Verification items for the finished model (mm, model axes). A direction names the side the tool comes from. Round coordinates to 2 decimals unless told otherwise and drop trailing zeros. Write each loop counter-clockwise with the first axis right and the second up, starting at its lowest first coordinate (ties: lowest second). Pieces come first, ordered by that corner, then holes.
from build123d import *

# Parameters (mm, degrees)
EXTRUDE_1_DEPTH     = 3
SKETCH_2_R          = 1.45
CUT_EXTRUDE_1_DEPTH = 3
SKETCH_3_W          = 50
SKETCH_3_H          = 3
EXTRUDE_2_DEPTH     = 8
SKETCH_4_W          = 50
SKETCH_4_H          = 5
EXTRUDE_3_DEPTH     = 16
SKETCH_6_W          = 27
SKETCH_6_H          = 5
EXTRUDE_4_DEPTH     = 7
SKETCH_7_R          = 1.45
CUT_EXTRUDE_2_DEPTH = 7
SKETCH_8_R          = 3
CUT_EXTRUDE_3_DEPTH = 2
FILLET_1_R          = 1
FILLET_2_R          = 2.5
SKETCH_9_R          = 1.45
CUT_EXTRUDE_4_DEPTH = 10


# Some blends are built 0.0001 mm under size
with BuildPart() as part:
    # Эскиз1 → Бобышка-Вытянуть1 (new body)
    with BuildSketch(Plane(origin=(0, 0, 0), x_dir=(1, 0, 0), z_dir=(0, 1, 0))):
        Polygon((-25, 0), (-12.5, 21.650635095), (12.5, 21.650635095), (25, 0), align=None)
    extrude(amount=EXTRUDE_1_DEPTH)

    # Эскиз2 → Вырез-Вытянуть1 (cut)
    with BuildSketch(Plane(origin=(0, 3, 0), x_dir=(1, 0, 0), z_dir=(0, 1, 0))):
        with Locations(Location((-10, 18.650635095, 0), (0, 0, 270))):
            Circle(SKETCH_2_R)
        with Locations(Location((-18, 4.794228634, 0), (0, 0, 270))):
            Circle(SKETCH_2_R)
        with Locations(Location((18, 4.794228634, 0), (0, 0, 90))):
            Circle(SKETCH_2_R)
        with Locations(Location((10, 18.650635095, 0), (0, 0, 90))):
            Circle(SKETCH_2_R)
        with Locations(Location((-6, 4.794228634, 0), (0, 0, 270))):
            Circle(SKETCH_2_R)
        with Locations(Location((6, 4.794228634, 0), (0, 0, 270))):
            Circle(SKETCH_2_R)
    extrude(amount=-CUT_EXTRUDE_1_DEPTH, mode=Mode.SUBTRACT)

    # Эскиз3 → Бобышка-Вытянуть2 (add)
    with BuildSketch(Plane.XY):
        with Locations((0, 1.5)):
            Rectangle(SKETCH_3_W, SKETCH_3_H)
    extrude(amount=EXTRUDE_2_DEPTH)

    # Эскиз4 → Бобышка-Вытянуть3 (add)
    with BuildSketch(Plane(origin=(0, 3, 0), x_dir=(1, 0, 0), z_dir=(0, 1, 0))):
        with Locations((0, -5.5)):
            Rectangle(SKETCH_4_W, SKETCH_4_H)
    extrude(amount=EXTRUDE_3_DEPTH)

    # Эскиз6 → Бобышка-Вытянуть4 (add)
    with BuildSketch(Plane.XY.offset(8)):
        with Locations((0, 3.5)):
            Rectangle(SKETCH_6_W, SKETCH_6_H)
    extrude(amount=EXTRUDE_4_DEPTH)

    # Эскиз7 → Вырез-Вытянуть2 (cut)
    with BuildSketch(Plane.XZ.offset(-1)):
        with Locations(Location((-8.5, 11.5, 0), (0, 0, 270))):
            Circle(SKETCH_7_R)
        with Locations(Location((8.5, 11.5, 0), (0, 0, 270))):
            Circle(SKETCH_7_R)
    extrude(amount=-CUT_EXTRUDE_2_DEPTH, mode=Mode.SUBTRACT)

    # Эскиз8 → Вырез-Вытянуть3 (cut)
    with BuildSketch(Plane.XZ.offset(-1)):
        with Locations(Location((-8.5, 11.5, 0), (0, 0, 270))):
            Circle(SKETCH_8_R)
        with Locations(Location((8.5, 11.5, 0), (0, 0, 270))):
            Circle(SKETCH_8_R)
    extrude(amount=-CUT_EXTRUDE_3_DEPTH, mode=Mode.SUBTRACT)

    # Скругление1
    fillet_1_edges = [part.edges().sort_by_distance(p)[0] for p in [
        (25, 9.5, 8),
        (-25, 9.5, 8),
        (0, 0, 8),
        (-25, 11, 3),
        (25, 11, 3),
    ]]
    fillet(fillet_1_edges, radius=FILLET_1_R - 0.0001)  # a hair under: the kernel refuses the full size

    # Скругление2
    # the kernel refuses this fillet: 2.5 mm, written as the material it takes off along each edge
    with BuildSketch(Plane(origin=(22.5, 2.5, 8), x_dir=(0, -1, 0), z_dir=(-1, 0, 0))) as fillet_2_piece_1:
        with BuildLine():
            CenterArc((1.5001, -0.9999), 0.9999, 0, 90)
            Line((2.5, -0.9999), (2.5, 0))
            Line((2.5, 0), (1.5001, 0))
        make_face()
    revolve(axis=Axis((22.5, 2.5, 8), (0, 0, 1)), revolution_arc=90, mode=Mode.SUBTRACT)
    with BuildSketch(Plane(origin=(-22.5, 2.5, 8), x_dir=(-1, 0, 0), z_dir=(0, 1, 0))) as fillet_2_piece_2:
        with BuildLine():
            CenterArc((1.5001, -0.9999), 0.9999, 0, 90)
            Line((2.5, -0.9999), (2.5, 0))
            Line((2.5, 0), (1.5001, 0))
        make_face()
    revolve(axis=Axis((-22.5, 2.5, 8), (0, 0, 1)), revolution_arc=90, mode=Mode.SUBTRACT)
    with BuildSketch(Plane(origin=(25, 0, -6.25), x_dir=(0, 1, 0), z_dir=(0, 0, 1))) as fillet_2_piece_3:
        with BuildLine():
            CenterArc((FILLET_2_R, FILLET_2_R), FILLET_2_R, 180, 90)
            Line((0, FILLET_2_R), (0, 0))
            Line((0, 0), (FILLET_2_R, 0))
        make_face()
    extrude(amount=14.25, mode=Mode.SUBTRACT)
    with BuildSketch(Plane(origin=(-25, 0, -6.25), x_dir=(0, 1, 0), z_dir=(0, 0, 1))) as fillet_2_piece_4:
        with BuildLine():
            CenterArc((FILLET_2_R, -FILLET_2_R), FILLET_2_R, 90, 90)
            Line((0, -FILLET_2_R), (0, 0))
            Line((0, 0), (FILLET_2_R, 0))
        make_face()
    extrude(amount=14.25, mode=Mode.SUBTRACT)
    with BuildSketch(Plane(origin=(-28.125, 0, 5.412658774), x_dir=(0, 1, 0), z_dir=(0.5000000000000041, 0, -0.8660254037844364)), Plane(origin=(-18.75, 0, -21.650635095), x_dir=(0, 1, 0), z_dir=(1, 0, 0)), Plane(origin=(9.375, 0, -27.063293868), x_dir=(0, 1, 0), z_dir=(0.5000000000000041, 0, 0.8660254037844364))) as fillet_2_piece_5:
        with BuildLine():
            CenterArc((FILLET_2_R, FILLET_2_R), FILLET_2_R, 180, 90)
            Line((0, FILLET_2_R), (0, 0))
            Line((0, 0), (FILLET_2_R, 0))
        make_face()
    extrude(amount=37.5, mode=Mode.SUBTRACT)

    # Эскиз9 → Вырез-Вытянуть4 (cut)
    with BuildSketch(Plane(origin=(0, 19, 0), x_dir=(1, 0, 0), z_dir=(0, 1, 0))):
        with Locations(Location((-18, -5.5, 0), (0, 0, 270))):
            Circle(SKETCH_9_R)
        with Locations(Location((18, -5.5, 0), (0, 0, 270))):
            Circle(SKETCH_9_R)
    extrude(amount=-CUT_EXTRUDE_4_DEPTH, mode=Mode.SUBTRACT)


solid = part.part
Q1. Depth check by flat-ended pin: P1, Ø5, axis at x = -8, z = 11, coming from the -Y side; P2, Ø4.5, axis at x = 18, z = -4.79, coming from the +Y side; P3, Ø2, axis at x = -1.5, z = 12.5, coming from the +Y side; P4, Ø3, axis at x = 4.5, y = 6.5, coming from the +Z side. Enter the tip coordinate at first touch or a pass-through.
Recorded:
P1: stops at y = 1
P2: stops at y = 3
P3: stops at y = 6
P4: stops at z = 15
Q2. Material ranges on line 1 along X through (y, z) = (16, 5.5); line 2 along X through (y, z) = (3.95, 11.5); line 3 along Z through (x, y) = (3, 17.75), recorded low to high.
Recorded:
line 1: x = -25 to -19.45, -16.55 to 16.55, 19.45 to 25
line 2: x = -13.5 to -9.95, -7.05 to 7.05, 9.95 to 13.5
line 3: z = 3 to 8
Q3. Tool access check on faces 4 (the flat face through (25, 11, 6)), 5 (the cylindrical face through (-6.47, 1.99, 13.71)), 6 (the cylindrical face through (17.12, 14.07, 4.35)), 7 (the cylindrical face through (-24.715, 11.112, 3.301)). Record the directions out of +Z, -Z, +X, -X, +Y, -Y that give a thin tool (end or side, any length) a straight path to the whole face; none if there is none.
Recorded:
face 4: +Z, -Z, +X, +Y, -Y
face 5: -Y
face 6: +Y
face 7: -Z, -X, +Y
Q4. Sectioned sample at B-B (y = 7). Enter the section's corners in (x, z), plus the area to 3 significant figures.
Recorded:
outline: (-25, 4) arc R1 ccw to (-24, 3) - (24, 3) arc R1 ccw to (25, 4) - (25, 7) arc R1 ccw to (24, 8) - (-24, 8) arc R1 ccw to (-25, 7) - close
area: 249 mm2
Q5. Release check for a two-part mould opening along X. For faces 1 (the flat face through (0, 6, 11)), 2 (the flat face through (13.5, 3, 11)), 3 (the cylindrical face through (-18.88, 14.07, 4.35)) record: released by +X, released by -X, zero draft, split by the parting line, or undercut.
Recorded:
face 1: zero draft
face 2: released by +X
face 3: undercut
Q6. Sectioned sample at A-A (z = 11.5). Enter the section's corners in (x, y), plus the area to 3 significant figures.
Recorded:
outline: (-13.5, 1) - (-11.5, 1) - (-11.5, 3) - (-9.95, 3) - (-9.95, 6) - (-13.5, 6) - close; (-7.05, 3) - (-5.5, 3) - (-5.5, 1) - (5.5, 1) - (5.5, 3) - (7.05, 3) - (7.05, 6) - (-7.05, 6) - close; (9.95, 3) - (11.5, 3) - (11.5, 1) - (13.5, 1) - (13.5, 6) - (9.95, 6) - close
area: 93.6 mm2
Q7. Sectioned sample at C-C (y = 17.5). Enter the section's corners in (x, z), plus the area to 3 significant figures.
Recorded:
outline: (-25, 4) arc R1 ccw to (-24, 3) - (24, 3) arc R1 ccw to (25, 4) - (25, 7) arc R1 ccw to (24, 8) - (-24, 8) arc R1 ccw to (-25, 7) - close; hole circle Ø2.9 at (-18, 5.5); hole circle Ø2.9 at (18, 5.5)
area: 236 mm2
